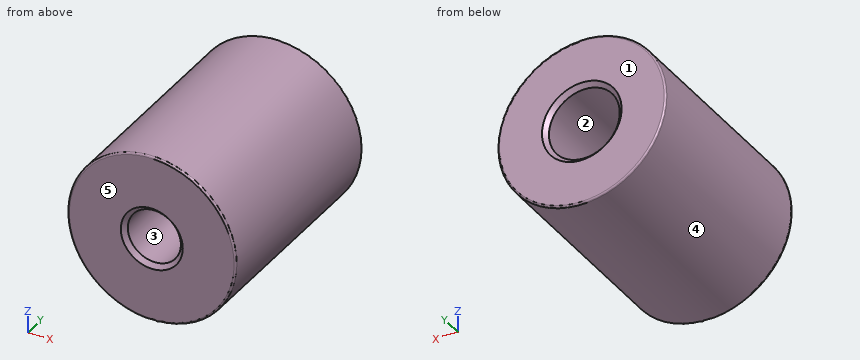
```python
from build123d import *

# Parameters (mm, degrees)
SKETCH_1_R          = 9.5
EXTRUDE_1_DEPTH     = 24.5
SKETCH_2_R          = 4
CUT_EXTRUDE_1_DEPTH = 16
SKETCH_3_R          = 3
CUT_EXTRUDE_2_DEPTH = 16
CHAMFER_1_SIZE      = 0.5
FILLET_1_R          = 0.2


with BuildPart() as part:
    # 草图1 → 凸台-拉伸1 (new body)
    with BuildSketch(Plane(origin=(0, 0, 0), x_dir=(1, 0, 0), z_dir=(0, 1, 0))):
        Circle(SKETCH_1_R)
    extrude(amount=EXTRUDE_1_DEPTH)

    # 草图2 → 切除-拉伸1 (cut)
    with BuildSketch(Plane(origin=(0, 24.5, 0), x_dir=(1, 0, 0), z_dir=(0, 1, 0))):
        Circle(SKETCH_2_R)
    extrude(amount=-CUT_EXTRUDE_1_DEPTH, mode=Mode.SUBTRACT)

    # 草图3 → 切除-拉伸2 (cut)
    with BuildSketch(Plane.XZ):
        Circle(SKETCH_3_R)
    extrude(amount=-CUT_EXTRUDE_2_DEPTH, mode=Mode.SUBTRACT)

    # 倒角1
    chamfer_1_edges = [part.edges().sort_by_distance(p)[0] for p in [
        (-3, 0, 0),
        (-4, 24.5, 0),
    ]]
    chamfer(chamfer_1_edges, length=CHAMFER_1_SIZE)

    # 圆角1
    fillet_1_edges = [part.edges().sort_by_distance(p)[0] for p in [
        (-9.5, 0, 0),
        (-9.5, 24.5, 0),
    ]]
    fillet(fillet_1_edges, radius=FILLET_1_R)


solid = part.part
```
Model file for the job. Use its own axes, mm. Face numbers are marked on the shaded views. A direction names the side the tool comes from. Coordinates: 2 decimals unless noted, no trailing zeros. Order: outer loops, then holes, each group sorted by start corner. A loop starts at its lowest first (then second) coordinate and runs counter-clockwise, first axis right, second up. Notation, with made-up numbers: (5.5, 35.25) -> (37.5, 35.25) arc R17 ccw to (37.5, 45.25) -> close; hole circle Ø8 at (-25.5, -8). An arc over 180 degrees is marked (long way). Answer as a JSON object with one key per item and string values. Group by question number.
1) Cut at A-A, the plane x = 0. Write the cut outline in (y, z), then the cut area to 3 significant figures.
2) Drill centre lines: L1, parallel to Z at x = 0, y = 19.5; L2, parallel to Z at x = 0, y = 4.75; L3, parallel to X at y = 4, z = -4. Where is each one in solid material? Low to high.
3) Flat gauge pins, fed straight in: pin 1 (8 mm diameter, centred on y = 7, z = -6.5, fed in from +X); pin 2 (6 mm diameter, centred on y = 21.5, z = -4.5, fed in from +X); pin 3 (10 mm diameter, centred on y = 5, z = -6.5, fed in from -X). Where does each tip first touch, or does it go through?
4) Pull direction Z, two halves, no side cores. Call the marked faces 3, 4 and 5: +Z half, -Z half, draft (parallel to the pull), parting line (faces both ways), or undercut.
5) Cut at B-B, the plane y = 6. Write the cut outline in (x, z), then the cut area to 3 significant figures.
6) Which spindle directions (+Z, -Z, +X, -X, +Y, -Y) get a long thin tool onto all of the face, cutting with end or side? Do the marked faces 1 and 2. Say none if no direction does.
7) Cut at C-C, the plane y = 22. Write the cut outline in (x, z).
Check values:
{
 "1": {"outline": "(0, -9.3) arc R0.2 ccw to (0.2, -9.5) -> (24.3, -9.5) arc R0.2 ccw to (24.5, -9.3) -> (24.5, -4.5) -> (24, -4) -> (8.5, -4) -> (8.5, -3) -> (0.5, -3) -> (0, -3.5) -> close; (0, 3.5) -> (0.5, 3) -> (8.5, 3) -> (8.5, 4) -> (24, 4) -> (24.5, 4.5) -> (24.5, 9.3) arc R0.2 ccw to (24.3, 9.5) -> (0.2, 9.5) arc R0.2 ccw to (0, 9.3) -> close", "area": "286 mm²"},
 "2": {"L1": "z = -9.5 to -4, 4 to 9.5", "L2": "z = -9.5 to -3, 3 to 9.5", "L3": "x = -8.62 to 8.62"},
 "3": {"pin 1": "stops at x = 9.17", "pin 2": "stops at x = 9.38", "pin 3": "stops at x = -9.38"},
 "4": {"face 3": "undercut", "face 4": "parting line", "face 5": "draft"},
 "5": {"outline": "circle Ø19 at (0, 0); hole circle Ø6 at (0, 0)", "area": "255 mm²"},
 "6": {"face 1": "+Z, -Z, +X, -X, +Y", "face 2": "+Y"},
 "7": {"outline": "circle Ø19 at (0, 0); hole circle Ø8 at (0, 0)"}
}
